```python
from build123d import *

# Parameters (mm, degrees)
SKETCH1_W              = 80
SKETCH1_H              = 80
PCB_DEPTH              = 2
SKETCH2_R              = 1.8
ATTACHMENT_HOLES_DEPTH = 3
LPATTERN1_COUNT        = 2
LPATTERN1_PITCH        = 70
LPATTERN1_COUNT_DIR2   = 2
LPATTERN1_PITCH_DIR2   = 70
IDUINO_DEPTH           = 10


with BuildPart() as part:
    # Sketch1 → PCB (new body)
    with BuildSketch(Plane(origin=(0, 0, 0), x_dir=(1, 0, 0), z_dir=(0, 1, 0))):
        with Locations((40, 40)):
            Rectangle(SKETCH1_W, SKETCH1_H)
    extrude(amount=PCB_DEPTH)

    # Sketch2 → Attachment Holes (cut, through all)
    with BuildSketch(Plane(origin=(0, 2, 0), x_dir=(1, 0, 0), z_dir=(0, 1, 0))):
        with Locations((5, 75)):
            Circle(SKETCH2_R)
    attachment_holes = extrude(amount=-ATTACHMENT_HOLES_DEPTH, mode=Mode.SUBTRACT)

    # LPattern1: Attachment Holes 2 × 2
    with Locations(*[(i * LPATTERN1_PITCH, 0, j * LPATTERN1_PITCH_DIR2) for i in range(LPATTERN1_COUNT) for j in range(LPATTERN1_COUNT_DIR2) if (i, j) != (0, 0)]):
        add(attachment_holes, mode=Mode.SUBTRACT)

    # Sketch3 → Iduino (add)
    with BuildSketch(Plane(origin=(0, 2, 0), x_dir=(1, 0, 0), z_dir=(0, 1, 0))):
        Polygon((-9, 28.800714626), (52.023315216, 89.824029842), (89.711939971, 52.135405088), (28.576534883, -9), align=None)
    extrude(amount=IDUINO_DEPTH)


solid = part.part
```
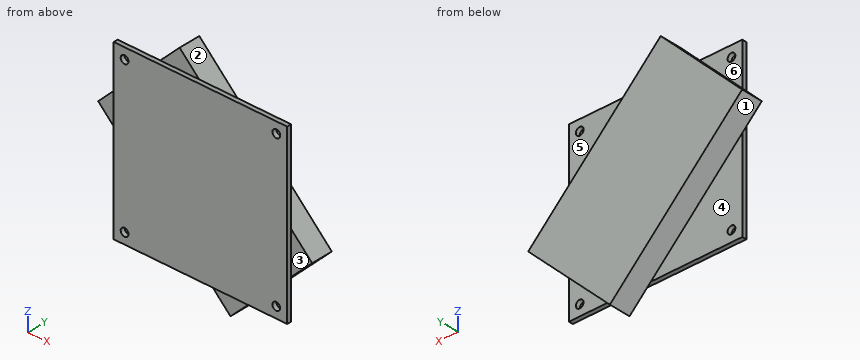
Could you check a few things on this model? Use its own coordinates, in mm. Face numbers are marked on the shaded views. A direction names the side the tool comes from. Coordinates: 2 decimals unless noted, no trailing zeros. Write each loop counter-clockwise with the first axis right and the second up, starting at its lowest first coordinate (ties: lowest second). Pieces come first, ordered by that corner, then holes. Notation, with made-up numbers: (80.5, 79) -> (119.5, 79) arc R11 cw to (119.5, 83) -> close; hole circle Ø5 at (88.5, 47). An arc over 180 degrees is marked (long way). One line per question, with ' | ' between items. Start each with the question number.
1. If we section it at A-A (z = -75): Please give me the cut outline in (x, y), and give its area (3 significant figures).
2. Please list where these lines run through material, in increasing order: line 1 along Z through (x, y) = (75, 1.05); line 2 along X through (y, z) = (0.7, -75); line 3 along Y through (x, z) = (72.5, -74.5).
3. If we section it at D-D (z = -25): Please give me the cut outline in (x, y), and give its area (3 significant figures).
4. Thinking about a two-plate mould opening in Z: for the marked faces 1, 2 and 3, which applies, pulls with the +Z half, pulls with the -Z half, needs draft (parallel to the pull), parting line crosses it, or undercut?
5. If we section it at C-C (y = 7.5): Please give me the cut outline in (x, z), and give its area (3 significant figures).
6. For the marked faces 4, 5 and 6, which set-ups out of +Z, -Z, +X, -X, +Y, -Y let a thin tool reach every point of the face, with its end or its side?
7. Will these pins go through, and if not, where does the flat tip stop? P1, Ø1.5, axis at y = 10, z = -69, coming from the -X side; P2, Ø3, axis at x = 40, y = 10, coming from the -Z side; P3, Ø0.6, axis at y = 1, z = -26, coming from the -X side.
8. If we section it at B-B (x = 5): Please give me the cut outline in (y, z).
Return value:
1) outline: (0, 0) -> (3.2, 0) -> (3.2, 2) -> (0, 2) -> close; (6.8, 0) -> (73.2, 0) -> (73.2, 2) -> (66.85, 2) -> (66.85, 12) -> (37.2, 12) -> (37.2, 2) -> (6.8, 2) -> close; (76.8, 0) -> (80, 0) -> (80, 2) -> (76.8, 2) -> close | area: 442 mm²
2) line 1: z = -80 to -76.8, -73.2 to -6.8, -3.2 to 0 | line 2: x = 0 to 3.2, 6.8 to 73.2, 76.8 to 80 | line 3: y = 0 to 2
3) outline: (-5.22, 2) -> (0, 2) -> (0, 0) -> (80, 0) -> (80, 2) -> (62.58, 2) -> (62.58, 12) -> (-5.22, 12) -> close | area: 838 mm²
4) face 1: pulls with the -Z half | face 2: pulls with the +Z half | face 3: needs draft
5) outline: (-9, -28.8) -> (52.02, -89.82) -> (89.71, -52.14) -> (28.58, 9) -> close | area: 4,600 mm²
6) face 4: -Z, -X, +Y | face 5: +Z, +X, +Y | face 6: +Z, -X, +Y
7) P1: stops at x = 30.45 | P2: stops at z = -79.3 | P3: stops at x = 0
8) outline: (0, -80) -> (2, -80) -> (2, -76.8) -> (0, -76.8) -> close; (0, -73.2) -> (2, -73.2) -> (2, -42.8) -> (12, -42.8) -> (12, -14.72) -> (2, -14.72) -> (2, -6.8) -> (0, -6.8) -> close; (0, -3.2) -> (2, -3.2) -> (2, 0) -> (0, 0) -> close
